Geometry check sheet. Reference: the model listing, model coordinates, mm. Round coordinates to 2 decimals unless told otherwise and drop trailing zeros. Write each loop counter-clockwise with the first axis right and the second up, starting at its lowest first coordinate (ties: lowest second). Pieces come first, ordered by that corner, then holes.
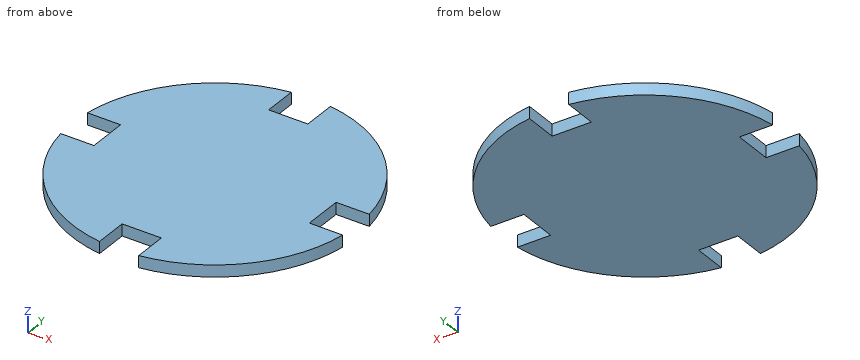
from build123d import *

# Parameters (mm, degrees)
BOSS_EXTRUDE1_DEPTH = 6.35


with BuildPart() as part:
    # Sketch1 → Boss-Extrude1 (new, symmetric)
    with BuildSketch(Plane.XY):
        with BuildLine():
            Line((150.946215587, -21), (115.332, -21))
            Line((115.332, -21), (115.332, 21))
            Line((115.332, 21), (150.946215587, 21))
            ThreePointArc((150.946215587, 21), (107.763073453, 107.763073453), (21, 150.946215587))
            Line((21, 150.946215587), (21, 115.332))
            Line((21, 115.332), (-21, 115.332))
            Line((-21, 115.332), (-21, 150.946215587))
            ThreePointArc((-21, 150.946215587), (-107.763073453, 107.763073453), (-150.946215587, 21))
            Line((-150.946215587, 21), (-115.332, 21))
            Line((-115.332, 21), (-115.332, -21))
            Line((-115.332, -21), (-150.946215587, -21))
            ThreePointArc((-150.946215587, -21), (-107.763073453, -107.763073453), (-21, -150.946215587))
            Line((-21, -150.946215587), (-21, -115.332))
            Line((-21, -115.332), (21, -115.332))
            Line((21, -115.332), (21, -150.946215587))
            ThreePointArc((21, -150.946215587), (107.763073453, -107.763073453), (150.946215587, -21))
        make_face()
    extrude(amount=BOSS_EXTRUDE1_DEPTH, both=True)


solid = part.part
1. Section check A-A (x = 130.5). Record the cut outline in (y, z).
2. Section check B-B (z = 3.75). Record the cut outline in (x, y), plus the area to 3 significant figures.
3. Section check C-C (y = -120.5). Record the cut outline in (x, z).
4. Scan lines: line 1 along X through (y, z) = (-8, -0.75); line 2 along Y through (x, z) = (127.5, 3.75). Record each from-to range of solid material in increasing order.
5. Depth check by flat-ended pin: pin 1 Ø4 at (y, z) = (135.5, -2.5) entering from -X; pin 2 Ø2 at (x, z) = (-112.5, 2) entering from -Y; pin 3 Ø2 at (y, z) = (-9, -5) entering from +X. Enter the tip coordinate at first touch or a pass-through.
6. Section check D-D (x = 4). Record the cut outline in (y, z), plus the area to 3 significant figures.
Results below:
1. outline: (-78.71, -6.35) - (-21, -6.35) - (-21, 6.35) - (-78.71, 6.35) - close; (21, -6.35) - (78.71, -6.35) - (78.71, 6.35) - (21, 6.35) - close
2. outline: (-150.95, -21) arc R152.4 ccw to (-21, -150.95) - (-21, -115.33) - (21, -115.33) - (21, -150.95) arc R152.4 ccw to (150.95, -21) - (115.33, -21) - (115.33, 21) - (150.95, 21) arc R152.4 ccw to (21, 150.95) - (21, 115.33) - (-21, 115.33) - (-21, 150.95) arc R152.4 ccw to (-150.95, 21) - (-115.33, 21) - (-115.33, -21) - close
2. area: 66,800 mm2
3. outline: (-93.3, -6.35) - (-21, -6.35) - (-21, 6.35) - (-93.3, 6.35) - close; (21, -6.35) - (93.3, -6.35) - (93.3, 6.35) - (21, 6.35) - close
4. line 1: x = -115.33 to 115.33
4. line 2: y = -83.48 to -21, 21 to 83.48
5. pin 1: stops at x = -73.51
5. pin 2: stops at y = -103.89
5. pin 3: stops at x = 115.33
6. outline: (-115.33, -6.35) - (115.33, -6.35) - (115.33, 6.35) - (-115.33, 6.35) - close
6. area: 2,930 mm2
